Input: dimensioned drawing with shaded views. Units: mm. Origin: part minimum x, y, z. Give positions to 0.01 mm unless a question says otherwise; leave off trailing zeros. Write each loop counter-clockwise with the first axis right and the second up, starting at its lowest first coordinate (ties: lowest second). Pieces come first, ordered by that corner, then holes. Notation, with made-up numbers: (-28.75, 16) -> (1.25, 16) arc R20 ccw to (1.25, 37) -> close; hole circle Ø3 at (70.5, 30). An arc over 180 degrees is marked (long way). Answer in a Markdown table with one row per item. Add a question column.
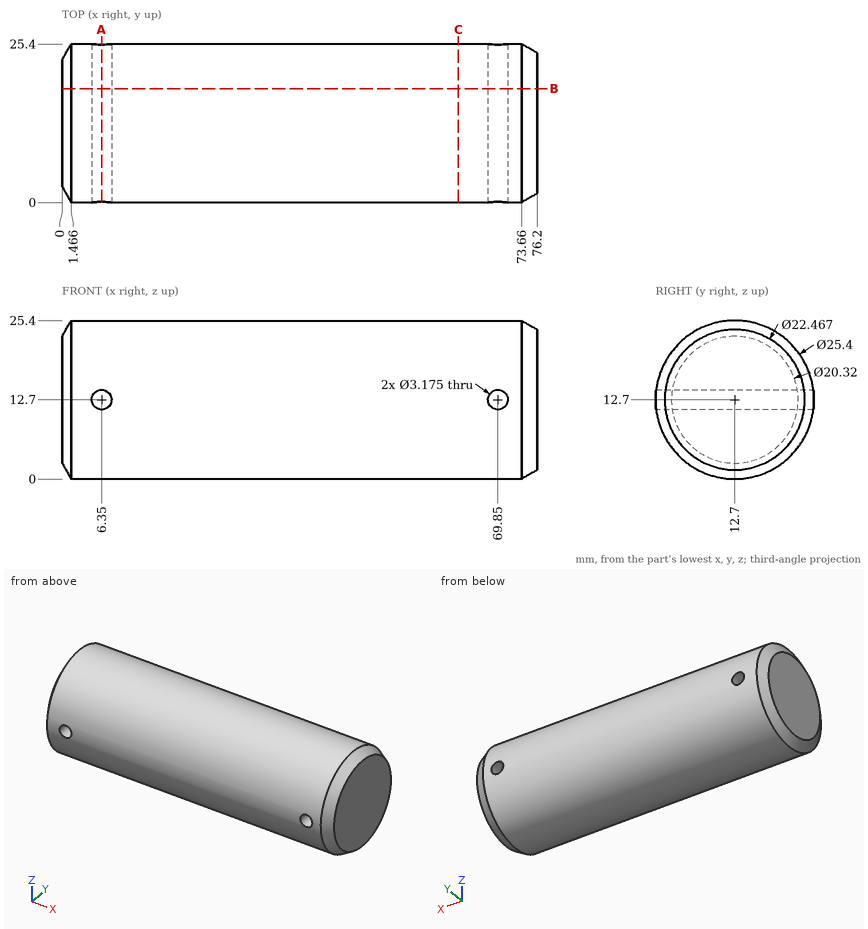
Q1. Section C-C on x = 63.5. Return loops of the section in (y, z).
Q2. Contact query for flat-ended pins moving along their axis: pin 1 Ø8 at (x, z) = (44, 22) entering from -Y; pin 2 Ø4 at (x, z) = (28, 5) entering from +Y; pin 3 Ø1.5 at (x, y) = (49.5, 8) entering from +Z; pin 4 Ø3 at (x, z) = (69.85, 12.7) entering from -Y. Output: stop coordinate, or through.
Q3. Line query: probe 1 along X at (y, z) = (16.75, 12.7); probe 2 along Z at (x, y) = (69, 16.5); probe 3 along Z at (x, y) = (25, 13). Output: solid intervals per line, ascending. Write a range as from..to.
Q4. Section B-B on y = 18.25. Count the separate pieces of the cut face and the enclosed holes in it, and give its area (3 significant figures).
Q5. Section A-A on x = 6.35. Return loops of the section in (y, z), and give its area (3 significant figures).
Checks:
| question | item | result |
|---|---|---|
| 1 | outline | circle Ø25.4 at (12.7, 12.7) |
| 2 | pin 1 | y = 1.16 |
| 2 | pin 2 | y = 24.05 |
| 2 | pin 3 | z = 24.77 |
| 2 | pin 4 | through |
| 3 | probe 1 | 0..4.76, 7.94..68.26, 71.44..76.2 |
| 3 | probe 2 | 0.58..11.36, 14.04..24.82 |
| 3 | probe 3 | 0..25.4 |
| 4 | separate pieces | 1 |
| 4 | enclosed holes | 2 |
| 4 | area | 1,720 mm^2 |
| 5 | outline | (0.1, 11.11) arc R12.7 ccw to (25.3, 11.11) -> close; (0.1, 14.29) -> (25.3, 14.29) arc R12.7 ccw to start |
| 5 | area | 426 mm^2 |
